The listing builds one solid part. Answer for the finished solid, in the listing's coordinates (mm). A direction names the side the tool comes from. Coordinates: 2 decimals unless noted, no trailing zeros. Write each loop counter-clockwise with the first axis right and the second up, starting at its lowest first coordinate (ties: lowest second). Pieces come first, ordered by that corner, then holes. Notation, with made-up numbers: M 16.25,9.25 L 73.25,9.25 A18 cw 73.25,25.25 Z; hole C 39,-34.5 d11. An arc over 180 degrees is marked long. Answer as CSV lines item,"result". Start each with the question number.
```python
from build123d import *

# Parameters (mm, degrees)
SKETCH1_R           = 14.475
BOSS_EXTRUDE1_DEPTH = 6.35
SKETCH2_R           = 2.75
CUT_EXTRUDE1_DEPTH  = 7.35
FILLET1_R           = 15


with BuildPart() as part:
    # Sketch1 → Boss-Extrude1 (new body)
    with BuildSketch(Plane(origin=(0, 0, 0), x_dir=(0, 0, -1), z_dir=(1, 0, 0))):
        with BuildLine():
            Line((-10, -22.912878475), (-10, -97.912878475))
            Line((-10, -97.912878475), (10, -97.912878475))
            Line((10, -97.912878475), (10, -22.912878475))
            ThreePointArc((10, -22.912878475), (0, 25), (-10, -22.912878475))
        make_face()
        Circle(SKETCH1_R, mode=Mode.SUBTRACT)
    extrude(amount=BOSS_EXTRUDE1_DEPTH)

    # Sketch2 → Cut-Extrude1 (cut, through all)
    with BuildSketch(Plane(origin=(6.35, 0, 0), x_dir=(0, 0, -1), z_dir=(1, 0, 0))):
        with Locations((0, -87.912878475)):
            Circle(SKETCH2_R)
        with Locations((0, -67.912878475)):
            Circle(SKETCH2_R)
        with Locations((0.431184648, -47.912878475)):
            Circle(SKETCH2_R)
    extrude(amount=-CUT_EXTRUDE1_DEPTH, mode=Mode.SUBTRACT)

    # Fillet1
    fillet1_edges = [part.edges().sort_by_distance(p)[0] for p in [
        (3.175, -22.912878475, 10),
        (3.175, -22.912878475, -10),
    ]]
    fillet(fillet1_edges, radius=FILLET1_R)


solid = part.part
```
1) Each of these flat-tipped pins is pushed along its axis until it touches: P1, Ø1, axis at x = 2.5, y = -32, coming from the -Z side; P2, Ø1.5, axis at x = 2.5, y = -68.5, coming from the +Z side; P3, Ø2, axis at y = -66, z = -3, coming from the -X side; P4, Ø1.5, axis at x = 2, z = 4.5, coming from the +Y side. Where does it stop, or does it pass through?
2) The part is cut by section C-C (x = 2.25). Determine the outline of the cut face in (y, z) (3 decimals), then the cut area to 3 significant figures.
3) The part is cut by section B-B (z = -7.5). Determine the outline of the cut face in (x, y), then the cut area to 3 significant figures.
4) Find the intervals of material crossed by line 1 (Y direction, x = 1.25, z = 0) (3 decimals); line 2 (Z direction, x = 3, y = -68); line 3 (Z direction, x = 6.25, y = -46.5), in increasing order. Write a range as from..to.
5) The part is cut by section A-A (y = 0). Determine the outline of the cut face in (x, z) (3 decimals), then the cut area to 3 significant figures.
6) The part is cut by section D-D (z = 0). Determine the outline of the cut face in (x, y) (3 decimals), then the cut area to 3 significant figures.
7) Which of the six approach directions +Z, -Z, +X, -X, +Y, -Y give full straight-line access (tool end or side, diameter ignored) to faces 1 (the face through (0, -22, 0)), 2 (the face through (3, -65, -10))?
8) For a pull along Z with two mould halves and no side action, classify faces 3 (the face through (3, -97.913, 0)), 4 (the face through (3.22, -50.6, 0.16)), 5 (the face through (3, -64, 10)) as +Z half, -Z half, draft (parallel to the pull), parting line (faces both ways), or undercut.
Completed:
1,P1,"z = -10"
1,P2,"z = 10"
1,P3,"x = 0"
1,P4,"y = 24.72"
2,outline,"M -97.913,-10 L -31.225,-10 A15 cw -19.516,-15.625 A25 ccw long -19.516,15.625 A15 cw -31.225,10 L -97.913,10 Z; hole C -87.913,0 d5.5; hole C -67.913,0 d5.5; hole C -47.913,-0.431 d5.5; hole C 0,0 d28.95"
2,area,"2,720 mm²"
3,outline,"M 0,-97.91 L 6.35,-97.91 L 6.35,-12.38 L 0,-12.38 Z; M 0,12.38 L 6.35,12.38 L 6.35,23.85 L 0,23.85 Z"
3,area,"616 mm²"
4,line 1,"-97.913..-90.663, -85.163..-70.663, -65.163..-50.629, -45.197..-14.475, 14.475..25"
4,line 2,"-10..-2.75, 2.75..10"
4,line 3,"-10..-2.79, 1.93..10"
5,outline,"M 0,-25 L 6.35,-25 L 6.35,-14.475 L 0,-14.475 Z; M 0,14.475 L 6.35,14.475 L 6.35,25 L 0,25 Z"
5,area,"134 mm²"
6,outline,"M 0,-97.913 L 6.35,-97.913 L 6.35,-90.663 L 0,-90.663 Z; M 0,-85.163 L 6.35,-85.163 L 6.35,-70.663 L 0,-70.663 Z; M 0,-65.163 L 6.35,-65.163 L 6.35,-50.629 L 0,-50.629 Z; M 0,-45.197 L 6.35,-45.197 L 6.35,-14.475 L 0,-14.475 Z; M 0,14.475 L 6.35,14.475 L 6.35,25 L 0,25 Z"
6,area,"492 mm²"
7,face 1,"+Z, -Z, -X, +Y, -Y"
7,face 2,"-Z, +X, -X, -Y"
8,face 3,"draft"
8,face 4,"undercut"
8,face 5,"+Z half"
